```python
from build123d import *

# Parameters (mm, degrees)
F0_W     = 73.845298
F0_H     = 76.810576
F1_DEPTH = 25.4
F2_R     = 19.363369
F3_DEPTH = 25.4
F5_DEPTH = 25.4


with BuildPart() as f1:
    # F0 (on Top) → F1 (new body)
    with BuildSketch(Plane.XY):
        Rectangle(F0_W, F0_H)
    extrude(amount=F1_DEPTH)

    # F2 (on face) → F3 (join)
    with BuildSketch(Plane.XY.offset(25.4)):
        Circle(F2_R)
    extrude(amount=F3_DEPTH)

    # F4 (on Front) → F5 (cut, symmetric)
    with BuildSketch(Plane.XZ):
        Polygon((20.831788, 68.200894), (-42.327017, 56.259107), (49.757458, 23.61821), align=None)
    extrude(amount=F5_DEPTH, both=True, mode=Mode.SUBTRACT)


solid = f1.part
```
Source: CAD feature listing. Evaluate the final solid. Frame: model axes, mm. A direction names the side the tool comes from. Give positions to 0.01 mm unless a question says otherwise; leave off trailing zeros. Write each loop counter-clockwise with the first axis right and the second up, starting at its lowest first coordinate (ties: lowest second). Pieces come first, ordered by that corner, then holes.
1. Section query B-B (x = -5). Return the cut outline in (y, z).
2. First-contact query: pin 1 (1 mm diameter, centred on x = -15, y = -2.5, fed in from +Z); pin 2 (22 mm diameter, centred on x = 1.5, y = -16.5, fed in from +Z); pin 3 (5 mm diameter, centred on x = 24.5, y = 0, fed in from +Z). Flat tips, straight axial feed; report the tip coordinate or a pass-through.
3. Section query C-C (z = 36). Return the cut outline in (x, y), then the cut area to 3 significant figures.
4. Section query D-D (x = 22.5). Return the cut outline in (y, z).
5. Access query for faces 1 (the face through (-9, 18, 25.4)), 2 (the face through (-0.27, -0.27, 41.35)). Directions: +Z, -Z, +X, -X, +Y, -Y. A direction counts if a zero-diameter tool reaches every point of the face in a straight line with its end or side. Return the directions, or none.
6. Section query A-A (y = 0). Return the cut outline in (x, z), then the cut area to 3 significant figures.
7. Material intervals for line 1 along Z through (x, y) = (-21, -19); line 2 along X through (y, z) = (-9.5, 28.5); line 3 along Y through (x, z) = (9, 38), sorted ascending.
Output values:
1. outline: (-38.41, 0) - (38.41, 0) - (38.41, 25.4) - (18.71, 25.4) - (18.71, 43.03) - (-18.71, 43.03) - (-18.71, 25.4) - (-38.41, 25.4) - close
2. pin 1: stops at z = 46.75
2. pin 2: stops at z = 44.62
2. pin 3: stops at z = 25.4
3. outline: (14.83, -12.45) - (14.83, 12.45) arc R19.36 ccw (long way) to start
3. area: 1,100 mm2
4. outline: (-38.41, 0) - (38.41, 0) - (38.41, 25.4) - (-38.41, 25.4) - close
5. face 1: +Z
5. face 2: +Z, +X, +Y, -Y
6. outline: (-36.92, 0) - (36.92, 0) - (36.92, 25.4) - (19.36, 25.4) - (19.36, 34.39) - (-19.36, 48.12) - (-19.36, 25.4) - (-36.92, 25.4) - close
6. area: 2,490 mm2
7. line 1: z = 0 to 25.4
7. line 2: x = -16.87 to 16.87
7. line 3: y = -17.14 to 17.14
